```python
from build123d import *

# Parameters (mm, degrees)
SKETCH_1_W          = 168
SKETCH_1_H          = 110
EXTRUDE_1_DEPTH     = 25
SKETCH_2_R          = 5.5
CUT_EXTRUDE_1_DEPTH = 203.358592602
SKETCH_3_W          = 86
SKETCH_3_H          = 55
EXTRUDE_2_DEPTH     = 132
SKETCH_4_R          = 31
CUT_EXTRUDE_2_DEPTH = 35
CHAMFER_1_SIZE      = 0.5
SKETCH_24_R         = 27
CUT_EXTRUDE_6_DEPTH = 18
SKETCH_25_R         = 31.5
CUT_EXTRUDE_7_DEPTH = 2
SKETCH_26_R         = 4
CUT_EXTRUDE_8_DEPTH = 21


with BuildPart() as part:
    # 草图1 → 凸台-拉伸1 (new body)
    with BuildSketch(Plane(origin=(0, 0, 0), x_dir=(1, 0, 0), z_dir=(0, 1, 0))):
        with Locations((84, 55)):
            Rectangle(SKETCH_1_W, SKETCH_1_H)
    extrude(amount=EXTRUDE_1_DEPTH)

    # 草图2 → 切除-拉伸1 (cut, through all)
    with BuildSketch(Plane(origin=(0, 25, 0), x_dir=(1, 0, 0), z_dir=(0, 1, 0))):
        with Locations(Location((15, 95, 0), (0, 0, 270))):
            Circle(SKETCH_2_R)
        with Locations(Location((153, 95, 0), (0, 0, 90))):
            Circle(SKETCH_2_R)
        with Locations(Location((153, 15, 0), (0, 0, 270))):
            Circle(SKETCH_2_R)
        with Locations(Location((15, 15, 0), (0, 0, 90))):
            Circle(SKETCH_2_R)
    extrude(amount=-CUT_EXTRUDE_1_DEPTH, mode=Mode.SUBTRACT)

    # 草图3 → 凸台-拉伸2 (add)
    with BuildSketch(Plane(origin=(0, 25, 0), x_dir=(1, 0, 0), z_dir=(0, 1, 0))):
        with Locations((84, 82.5)):
            Rectangle(SKETCH_3_W, SKETCH_3_H)
    extrude(amount=EXTRUDE_2_DEPTH)

    # 草图4 → 切除-拉伸2 (cut)
    with BuildSketch(Plane.XY.offset(-55)):
        with Locations((84, 106)):
            Circle(SKETCH_4_R)
    extrude(amount=-CUT_EXTRUDE_2_DEPTH, mode=Mode.SUBTRACT)

    # 倒角1
    chamfer_1_edges = [part.edges().sort_by_distance(p)[0] for p in [
        (53, 106, -55),
    ]]
    chamfer(chamfer_1_edges, length=CHAMFER_1_SIZE)

    # 草图24 → 切除-拉伸6 (cut)
    with BuildSketch(Plane(origin=(0, 0, -110), x_dir=(-1, 0, 0), z_dir=(0, 0, -1))):
        with Locations((-84, 106)):
            Circle(SKETCH_24_R)
    extrude(amount=-CUT_EXTRUDE_6_DEPTH, mode=Mode.SUBTRACT)

    # 草图25 → 切除-拉伸7 (cut)
    with BuildSketch(Plane(origin=(0, 0, -92), x_dir=(-1, 0, 0), z_dir=(0, 0, -1))):
        with Locations((-84, 106)):
            Circle(SKETCH_25_R)
    extrude(amount=-CUT_EXTRUDE_7_DEPTH, mode=Mode.SUBTRACT)

    # 草图26 → 切除-拉伸8 (cut)
    with BuildSketch(Plane.XY.offset(-55)):
        with Locations((84, 147)):
            Circle(SKETCH_26_R)
        with Locations((119.507041555, 126.5)):
            Circle(SKETCH_26_R)
        with Locations((119.507041555, 85.5)):
            Circle(SKETCH_26_R)
        with Locations((84, 65)):
            Circle(SKETCH_26_R)
        with Locations((48.492958445, 85.5)):
            Circle(SKETCH_26_R)
        with Locations((48.492958445, 126.5)):
            Circle(SKETCH_26_R)
    extrude(amount=-CUT_EXTRUDE_8_DEPTH, mode=Mode.SUBTRACT)


solid = part.part
```
Input: part model. Units: mm. Frame: model coordinates. A direction names the side the tool comes from. Round coordinates to 2 decimals unless told otherwise and drop trailing zeros. Loops run counter-clockwise (first coordinate to the right, second up) from the corner with the lowest first, then second, coordinate; pieces in that order, holes last. Notation, with made-up numbers: (65.25, -25) -> (80.25, -25) arc R26 ccw to (80.25, -10) -> close; hole circle Ø7 at (-16.5, 33). An arc over 180 degrees is marked (long way). One line per item, written item: value.
(1) Mould query, pull axis Z, two halves, no side actions, for faces 1 (the face through (83, 60, -110)), 2 (the face through (83.133, 61.095, -65.353)), 3 (the face through (63.1, 82.8, -90)). Classes: pulls with the +Z half, pulls with the -Z half, needs draft (parallel to the pull), parting line crosses it, or undercut.
Geometry check:
face 1: pulls with the -Z half
face 2: needs draft
face 3: undercut
(2) Material intervals for line 1 (Y direction, x = 84, z = -77); line 2 (Y direction, x = 91.5, z = -72.5); line 3 (Y direction, x = 86.5, z = -59), sorted ascending. Write a range as [from, to].
Geometry check:
line 1: [0, 75], [137, 157]
line 2: [0, 75.92], [136.08, 157]
line 3: [0, 61.88], [68.12, 75.1], [136.9, 143.88], [150.12, 157]
(3) Pin query (flat end, axial travel): pin 1 (5 mm diameter, centred on y = 89, z = -85.5, fed in from +X); pin 2 (4 mm diameter, centred on x = 85.5, y = 66.5, fed in from +Z); pin 3 (1 mm diameter, centred on x = 110, z = -40, fed in from +Y). Return the tip coordinate at first contact, or that it passes through.
Geometry check:
pin 1: x = 127
pin 2: z = -55
pin 3: y = 25
(4) Section B-B (y = 106). Return the cut outline in (x, z).
Geometry check:
outline: (41, -110) -> (57, -110) -> (57, -92) -> (52.5, -92) -> (52.5, -90) -> (53, -90) -> (53, -55.5) -> (52.5, -55) -> (41, -55) -> close; (111, -110) -> (127, -110) -> (127, -55) -> (115.5, -55) -> (115, -55.5) -> (115, -90) -> (115.5, -90) -> (115.5, -92) -> (111, -92) -> close
(5) Section C-C (z = -15). Return the cut outline in (x, y), plus the area to 3 significant figures.
Geometry check:
outline: (0, 0) -> (9.5, 0) -> (9.5, 25) -> (0, 25) -> close; (20.5, 0) -> (147.5, 0) -> (147.5, 25) -> (20.5, 25) -> close; (158.5, 0) -> (168, 0) -> (168, 25) -> (158.5, 25) -> close
area: 3,650 mm2
(6) Section A-A (z = -95). Return the cut outline in (x, y), plus the area to 3 significant figures.
Geometry check:
outline: (0, 0) -> (9.5, 0) -> (9.5, 25) -> (0, 25) -> close; (20.5, 0) -> (147.5, 0) -> (147.5, 25) -> (127, 25) -> (127, 157) -> (41, 157) -> (41, 25) -> (20.5, 25) -> close; (158.5, 0) -> (168, 0) -> (168, 25) -> (158.5, 25) -> close; hole circle Ø54 at (84, 106)
area: 12,700 mm2
(7) Section D-D (x = 15). Return the cut outline in (y, z), plus the area to 3 significant figures.
Geometry check:
outline: (0, -110) -> (25, -110) -> (25, -100.5) -> (0, -100.5) -> close; (0, -89.5) -> (25, -89.5) -> (25, -20.5) -> (0, -20.5) -> close; (0, -9.5) -> (25, -9.5) -> (25, 0) -> (0, 0) -> close
area: 2,200 mm2
(8) Set-up query: faces 4 (the face through (121.66, 129.87, -65.35)), 5 (the face through (107.217, 127.289, -91.014)), 6 (the face through (83, 157, -83)), 7 (the face through (41, 90, -82)), 8 (the face through (83, 25, -44)). Return all of +Z, -Z, +X, -X, +Y, -Y with unobstructed straight access to the full face (end or side cutting, diameter ignored); none if empty.
Geometry check:
face 4: +Z
face 5: none
face 6: +Z, -Z, +X, -X, +Y
face 7: +Z, -Z, -X, +Y
face 8: +Z, +Y
